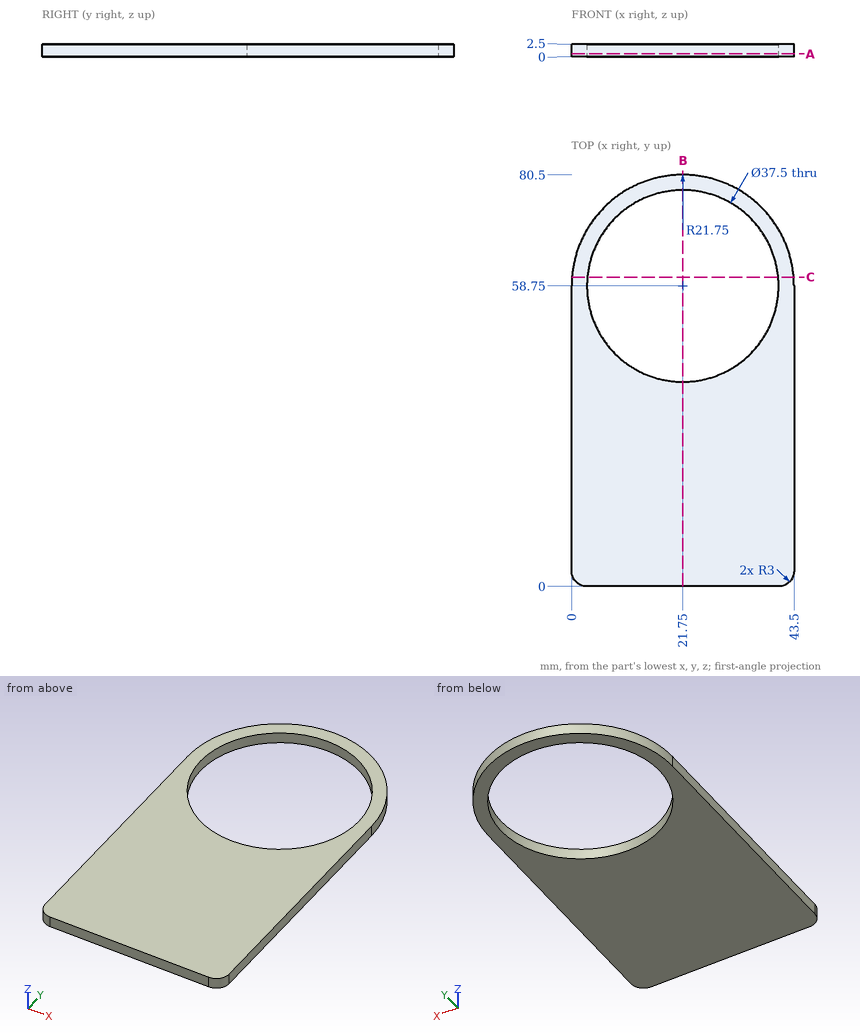
Can you work these out from the drawing? Everything is in mm from the part's minimum corner. Round coordinates to 2 decimals unless told otherwise and drop trailing zeros. Loops run counter-clockwise (first coordinate to the right, second up) from the corner with the lowest first, then second, coordinate; pieces in that order, holes last. Notation, with made-up numbers: (23, 65.25) -> (31, 65.25) arc R23 ccw to (31, 90.25) -> close; hole circle Ø5 at (-31.75, -32). An arc over 180 degrees is marked (long way). One line per question, with ' | ' between items.
(1) If we section it at A-A on z = 0.55: List the corners of the cut face in (x, y) for me, and give its area (3 significant figures).
Model answer:
outline: (0, 3) arc R3 ccw to (3, 0) -> (40.5, 0) arc R3 ccw to (43.5, 3) -> (43.5, 58.75) arc R21.75 ccw to (0, 58.75) -> close; hole circle Ø37.5 at (21.75, 58.75) | area: 2,190 mm^2
(2) If we section it at C-C on y = 60.5: List the corners of the cut face in (x, z) for me, and give its area (3 significant figures).
Model answer:
outline: (0.07, 0) -> (3.08, 0) -> (3.08, 2.5) -> (0.07, 2.5) -> close; (40.42, 0) -> (43.43, 0) -> (43.43, 2.5) -> (40.42, 2.5) -> close | area: 15.1 mm^2
(3) If we section it at B-B on x = 21.75: List the corners of the cut face in (y, z) for me.
Model answer:
outline: (0, 0) -> (40, 0) -> (40, 2.5) -> (0, 2.5) -> close; (77.5, 0) -> (80.5, 0) -> (80.5, 2.5) -> (77.5, 2.5) -> close
(4) If I drill on probe 1 along X at (y, z) = (58, 0.1) (3 decimals); probe 2 along Y at (x, z) = (21.75, 1.6); probe 3 along Y at (x, z) = (38, 0.8), over which ranges is the centre line in solid material (lowest first)?
Model answer:
probe 1: x = 0 to 3.015, 40.485 to 43.5 | probe 2: y = 0 to 40, 77.5 to 80.5 | probe 3: y = 0 to 49.4, 68.1 to 73.21
